Input: part model. Units: mm. Frame: model coordinates. Coordinates: 2 decimals unless noted, no trailing zeros. Loops run counter-clockwise (first coordinate to the right, second up) from the corner with the lowest first, then second, coordinate; pieces in that order, holes last. Notation, with made-up numbers: (61.5, 10.25) - (71.5, 10.25) arc R7 ccw to (71.5, 20.25) - close; hole circle Ø9 at (-7.5, 68). An arc over 180 degrees is marked (long way). Use one line per item in the form item = value.
from build123d import *

# Parameters (mm, degrees)
SKETCH11_R                          = 3.4
SKETCH11_W                          = 3.75
SKETCH11_H                          = 3.75
F_3030_3030_PROFILE_ZYLTECH_1_DEPTH = 325.999796


with BuildPart() as part:
    # Sketch11 → 3030 3030 PROFILE ZYLTECH(1) (new body)
    with BuildSketch(Plane(origin=(0, 0, 162.999898), x_dir=(1, 0, 0), z_dir=(0, 0, -1))):
        with BuildLine():
            Line((-9.805634919, -8.25), (-5.8, -4.244365081))
            Line((-5.8, -4.244365081), (-5.8, 4.244365081))
            Line((-5.8, 4.244365081), (-9.805634919, 8.25))
            Line((-9.805634919, 8.25), (-13, 8.25))
            Line((-13, 8.25), (-13, 4.07))
            Line((-13, 4.07), (-15, 4.07))
            Line((-15, 4.07), (-15, 12.5))
            ThreePointArc((-15, 12.5), (-14.267766953, 14.267766953), (-12.5, 15))
            Line((-12.5, 15), (-4.07, 15))
            Line((-4.07, 15), (-4.07, 13))
            Line((-4.07, 13), (-8.25, 13))
            Line((-8.25, 13), (-8.25, 9.805634919))
            Line((-8.25, 9.805634919), (-4.244365081, 5.8))
            Line((-4.244365081, 5.8), (4.244365081, 5.8))
            Line((4.244365081, 5.8), (8.25, 9.805634919))
            Line((8.25, 9.805634919), (8.25, 13))
            Line((8.25, 13), (4.07, 13))
            Line((4.07, 13), (4.07, 15))
            Line((4.07, 15), (12.5, 15))
            ThreePointArc((12.5, 15), (14.267766953, 14.267766953), (15, 12.5))
            Line((15, 12.5), (15, 4.07))
            Line((15, 4.07), (13, 4.07))
            Line((13, 4.07), (13, 8.25))
            Line((13, 8.25), (9.805634919, 8.25))
            Line((9.805634919, 8.25), (5.8, 4.244365081))
            Line((5.8, 4.244365081), (5.8, -4.244365081))
            Line((5.8, -4.244365081), (9.805634919, -8.25))
            Line((9.805634919, -8.25), (13, -8.25))
            Line((13, -8.25), (13, -4.07))
            Line((13, -4.07), (15, -4.07))
            Line((15, -4.07), (15, -12.5))
            ThreePointArc((15, -12.5), (14.267766953, -14.267766953), (12.5, -15))
            Line((12.5, -15), (4.07, -15))
            Line((4.07, -15), (4.07, -13))
            Line((4.07, -13), (8.25, -13))
            Line((8.25, -13), (8.25, -9.805634919))
            Line((8.25, -9.805634919), (4.244365081, -5.8))
            Line((4.244365081, -5.8), (-4.244365081, -5.8))
            Line((-4.244365081, -5.8), (-8.25, -9.805634919))
            Line((-8.25, -9.805634919), (-8.25, -13))
            Line((-8.25, -13), (-4.07, -13))
            Line((-4.07, -13), (-4.07, -15))
            Line((-4.07, -15), (-12.5, -15))
            ThreePointArc((-12.5, -15), (-14.267766953, -14.267766953), (-15, -12.5))
            Line((-15, -12.5), (-15, -4.07))
            Line((-15, -4.07), (-13, -4.07))
            Line((-13, -4.07), (-13, -8.25))
            Line((-13, -8.25), (-9.805634919, -8.25))
        make_face()
        Circle(SKETCH11_R, mode=Mode.SUBTRACT)
        with Locations((-11.625, 11.625)):
            Rectangle(SKETCH11_W, SKETCH11_H, mode=Mode.SUBTRACT)
        with Locations((11.625, 11.625)):
            Rectangle(SKETCH11_W, SKETCH11_H, mode=Mode.SUBTRACT)
        with Locations((-11.625, -11.625)):
            Rectangle(SKETCH11_W, SKETCH11_H, mode=Mode.SUBTRACT)
        with Locations((11.625, -11.625)):
            Rectangle(SKETCH11_W, SKETCH11_H, mode=Mode.SUBTRACT)
    extrude(amount=F_3030_3030_PROFILE_ZYLTECH_1_DEPTH)


solid = part.part
Q1. Cut plane A-A, the plane y = 0. Return loops of the section in (x, z).
Check values:
outline = (-5.8, -163) - (-3.4, -163) - (-3.4, 163) - (-5.8, 163) - close; (3.4, -163) - (5.8, -163) - (5.8, 163) - (3.4, 163) - close
Q2. Pull-direction query (X, two-part tool) for faces 1 (the flat face through (15, -8, 2)), 2 (the flat face through (0, -5.8, 2)), 3 (the flat face through (-8, -15, 2)); classes: pulls with the +X half, pulls with the -X half, needs draft (parallel to the pull), parting line crosses it, or undercut.
Check values:
face_1 = pulls with the +X half
face_2 = undercut
face_3 = needs draft
Q3. First-contact query: P1, Ø3, axis at x = 2.5, z = 28, coming from the +Y side; P2, Ø0.6, axis at y = 14, z = -19.5, coming from the +X side; P3, Ø0.6, axis at y = -14, z = 56, coming from the -X side. Flat tips, straight axial feed; report the tip coordinate or a pass-through.
Check values:
P1 = 5.8
P2 = 14.69
P3 = -14.69
Q4. Cut plane C-C, the plane z = -87.5. Give the number of separate pieces and of enclosed holes in the cut face, then the cut area to 3 significant figures.
Check values:
separate_pieces = 1
enclosed_holes = 5
area = 326 mm²
Q5. Ray query, line 1 along Y through (x, z) = (10, 119.5); line 2 along X through (y, z) = (7.75, -135.5). Return the intervals inside material, ascending. Write a range as [from, to].
Check values:
line_1 = [-15, -13.5], [-9.75, -8.25], [8.25, 9.75], [13.5, 15]
line_2 = [-15, -13], [-9.31, -6.19], [6.19, 9.31], [13, 15]
